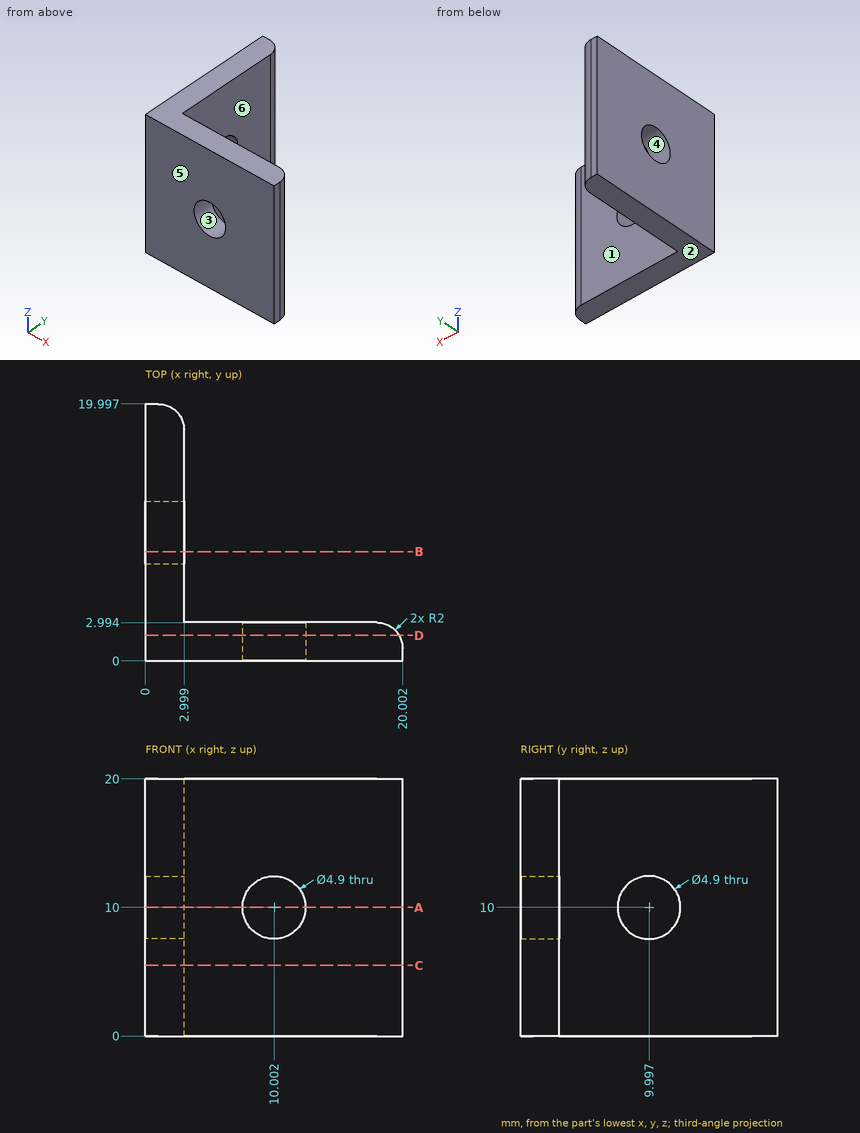
Drawing for the job (mm, zero at the part's lowest x, y, z). A direction names the side the tool comes from. Give positions to 0.01 mm unless a question says otherwise; leave off trailing zeros. Write each loop counter-clockwise with the first axis right and the second up, starting at its lowest first coordinate (ties: lowest second). Pieces come first, ordered by that corner, then holes. Notation, with made-up numbers: (6, 87.5) -> (33, 87.5) arc R14 ccw to (33, 99.5) -> close; hole circle Ø10 at (-15, 69.5). An arc over 180 degrees is marked (long way). Put each result on its own line as item: value. Start each with the question number.
Item 1: Wall check: L1, parallel to Y at x = 0.75, z = 10; L2, parallel to Y at x = 8, z = 13.25 (1 decimal); L3, parallel to X at y = 2.35, z = 10. Give the ranges that are in metal, low to high. Write a range as [from, to].
Item 2: Pin check, flat tips, straight feed: pin 1 Ø4 at (x, y) = (17, 6.5) entering from -Z; pin 2 Ø5.5 at (y, z) = (10, 10) entering from +X; pin 3 Ø5.5 at (x, z) = (10, 10) entering from +Y; pin 4 Ø6 at (x, y) = (12.5, 4) entering from -Z. Stop position of each tip, or through.
Item 3: Cut at A-A (z = 10). List the corners of the cut face in (x, y) (1 decimal).
Item 4: Cut at C-C (z = 5.5). List the corners of the cut face in (x, y) (1 decimal).
Item 5: Which spindle directions (+Z, -Z, +X, -X, +Y, -Y) get a long thin tool onto all of the face, cutting with end or side? Do the marked faces 5 and 6. Say none if no direction does.
Item 6: Cut at D-D (y = 2). List the corners of the cut face in (x, z), then the cut area to 3 significant figures.
Item 7: Pull direction Z, two halves, no side cores. Call the marked faces 1, 2, 3 and 4: pulls with the +Z half, pulls with the -Z half, needs draft (parallel to the pull), parting line crosses it, or undercut.
Item 8: Cut at B-B (y = 8.5). List the corners of the cut face in (x, z).
Answer list:
1. L1: y = [0, 7.55], [12.45, 20]
1. L2: y = [0, 3]
1. L3: x = [0, 7.55], [12.45, 19.47]
2. pin 1: passes through
2. pin 2: stops at x = 3
2. pin 3: stops at y = 2.99
2. pin 4: stops at z = 0
3. outline: (0, 0) -> (7.6, 0) -> (7.6, 3) -> (3, 3) -> (3, 7.5) -> (0, 7.5) -> close; (0, 12.4) -> (3, 12.4) -> (3, 18) arc R2 ccw to (1, 20) -> (0, 20) -> close; (12.5, 0) -> (20, 0) -> (20, 1) arc R2 ccw to (18, 3) -> (12.5, 3) -> close
4. outline: (0, 0) -> (20, 0) -> (20, 1) arc R2 ccw to (18, 3) -> (3, 3) -> (3, 18) arc R2 ccw to (1, 20) -> (0, 20) -> close
5. face 5: +Z, -Z, +X, -X, -Y
5. face 6: +Z, -Z, +X, +Y
6. outline: (0, 0) -> (19.73, 0) -> (19.73, 20) -> (0, 20) -> close; hole circle Ø4.9 at (10, 10)
6. area: 376 mm2
7. face 1: needs draft
7. face 2: pulls with the -Z half
7. face 3: undercut
7. face 4: undercut
8. outline: (0, 0) -> (3, 0) -> (3, 8.06) -> (0, 8.06) -> close; (0, 11.94) -> (3, 11.94) -> (3, 20) -> (0, 20) -> close
